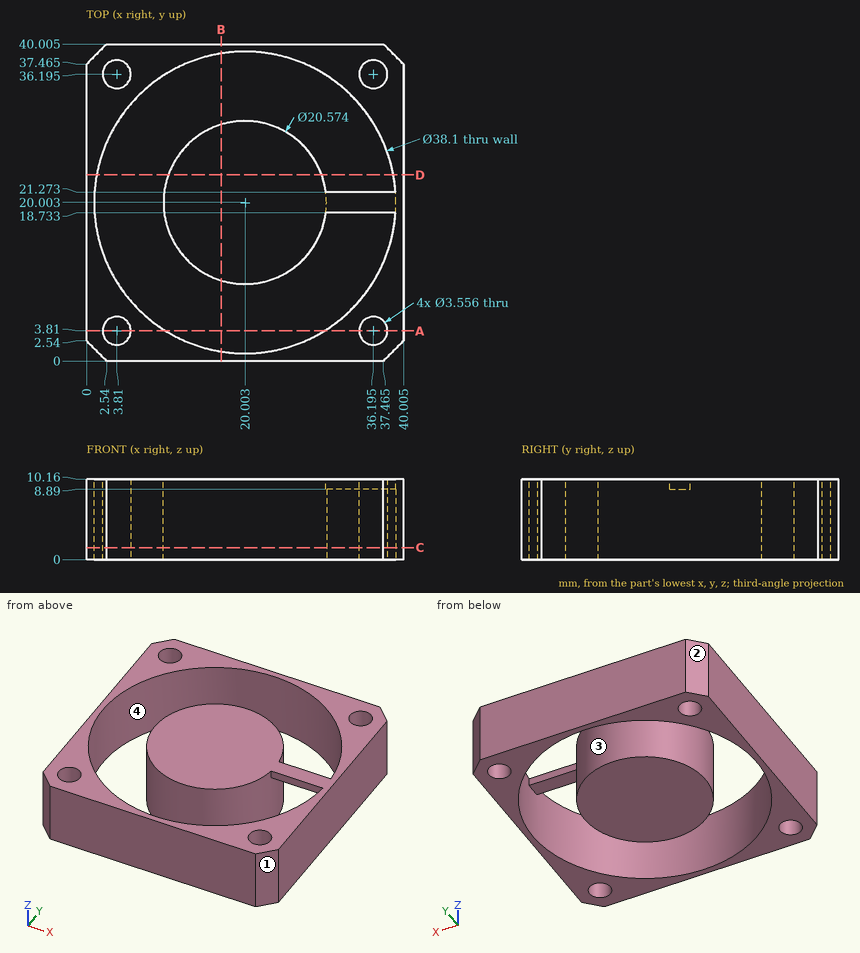
For this review, use the dimensioned drawing (mm, ordinates from the lowest corner) and the shaded views. Give positions to 0.01 mm unless a question says otherwise; leave off trailing zeros. Write each loop counter-clockwise with the first axis right and the second up, starting at its lowest first coordinate (ties: lowest second). Pieces come first, ordered by that corner, then holes. Notation, with made-up numbers: M 82,21.5 L 109,21.5 A31 ccw 109,57.5 Z; hole C 3.25,14 d7. An arc over 180 degrees is marked long. Answer as a JSON object with one key per item and string values. Group by question number.
Item 1: Draft analysis for pull direction X (two halves, no side actions). For the marked faces 1, 2, 3 and 4, state which applies: +X half, -X half, draft (parallel to the pull), parting line (faces both ways), or undercut.
Item 2: Consider section C-C on z = 1.5. Count the separate pieces of the cut face and the enclosed holes in it.
Item 3: For probe 1 along Y at (x, z) = (5, 1.5) (1 decimal); probe 2 along Y at (x, z) = (4, 7) (1 decimal); probe 3 along X at (y, z) = (37.5, 9) (1 decimal), list the stretches that pass through material, from the lowest coordinate up. Write a range as [from, to].
Item 4: Consider section B-B on x = 17. Write out the cut boundary in (y, z) (1 decimal).
Item 5: Consider section D-D on y = 23.5. Write out the cut boundary in (x, z) (1 decimal).
Item 6: For pin 1 Ø0.8 at (x, y) = (32.5, 19.5) entering from -Z, flat-tipped, find the tip position at first contact; note if it passes through.
Item 7: Consider section A-A on y = 3.81. Write out the cut boundary in (x, z) (1 decimal), plus the area to 3 significant figures.
Check result:
{
 "1": {"face 1": "+X half", "face 2": "-X half", "face 3": "undercut", "face 4": "undercut"},
 "2": {"separate pieces": "2", "enclosed holes": "5"},
 "3": {"probe 1": "y = [0, 2.5], [5.1, 8.3], [31.7, 34.9], [37.5, 40]", "probe 2": "y = [0, 2], [5.6, 9.7], [30.3, 34.4], [38, 40]", "probe 3": "x = [0, 2.6], [5, 12.5], [27.5, 35], [37.4, 40]"},
 "4": {"outline": "M 0,0 L 1.2,0 L 1.2,10.2 L 0,10.2 Z; M 10.2,0 L 29.8,0 L 29.8,10.2 L 10.2,10.2 Z; M 38.8,0 L 40,0 L 40,10.2 L 38.8,10.2 Z"},
 "5": {"outline": "M 0,0 L 1.3,0 L 1.3,10.2 L 0,10.2 Z; M 10.3,0 L 29.7,0 L 29.7,10.2 L 10.3,10.2 Z; M 38.7,0 L 40,0 L 40,10.2 L 38.7,10.2 Z"},
 "6": {"pin 1": "stops at z = 8.89"},
 "7": {"outline": "M 0,0 L 2,0 L 2,10.2 L 0,10.2 Z; M 5.6,0 L 10,0 L 10,10.2 L 5.6,10.2 Z; M 30,0 L 34.4,0 L 34.4,10.2 L 30,10.2 Z; M 38,0 L 40,0 L 40,10.2 L 38,10.2 Z", "area": "130 mm^2"}
}
